Read the model definition and answer for the solid it produces. Units are mm, in the model's axes. A direction names the side the tool comes from. Give positions to 0.01 mm unless a question says otherwise; leave off trailing zeros. Write each loop counter-clockwise with the first axis right and the second up, starting at its lowest first coordinate (ties: lowest second). Pieces come first, ordered by that corner, then holes. Notation, with made-up numbers: M 47.5,43.5 L 80.5,43.5 A20 ccw 80.5,54.5 Z; hole C 55,67 d4. An arc over 180 degrees is marked long. Use a Markdown table: item, result. Add a question column.
Item 1: A cutting plane is placed at B-B on y = -7.5. Determine the outline of the cut face in (x, z), then the cut area to 3 significant figures.
Item 2: A cutting plane is placed at C-C on x = 19. Determine the outline of the cut face in (y, z), then the cut area to 3 significant figures.
Item 3: A cutting plane is placed at A-A on z = 34. Determine the outline of the cut face in (x, y), then the cut area to 3 significant figures.
Item 4: Consider probe 1 along Y at (x, z) = (-1, 11); probe 2 along Z at (x, y) = (9.5, -5); probe 3 along Y at (x, z) = (11.5, 16). Determine where each line is inside the solid, lowest interval first. Write a range as [from, to].
Item 5: Given P1, Ø13.5, axis at x = 33.5, z = -1.5, coming from the -Y side; P2, Ø9, axis at y = 40, z = -5, coming from the +X side; P3, Ø2, axis at x = 12, z = 51.5, coming from the -Y side; P4, Ø8, axis at x = 29, z = 48.5, coming from the -Y side, each flat-ended and moving along its own axis, determine where each tip first touches the part or whether it passes through.
Item 6: For faces 1 (the flat face through (32, 0, 2)), 2 (the flat face through (0, 0, 63.5)), 3 (the flat face through (0, 34, 1)), determine the directions among +Z, -Z, +X, -X, +Y, -Y from which every point of the face is accessible in a straight line to the end or side of a thin tool.
from build123d import *

# Parameters (mm, degrees)
F0_R     = 21.5573937043
F1_DEPTH = 63.5
F3_DEPTH = 1.778
F5_DEPTH = 1.27


with BuildPart() as f1:
    # F0 (on Top) → F1 (new body)
    with BuildSketch(Plane.XY):
        Circle(F0_R)
    extrude(amount=F1_DEPTH)

    # F2 (on Right) → F3 (join)
    with BuildSketch(Plane.YZ):
        with BuildLine():
            add(Edge.make_bspline(
                [(21.4230585843, 18.8257303089), (25.4152571812, 17.7337542467), (35.0627733159, 15.0948933727), (62.3459313723, -26.3349238901), (35.309978925, -8.8714455783), (21.5757172555, 0)],
                knots=[0, 0, 0, 0, 0.257781652, 0.6229531389, 1, 1, 1, 1], degree=3))
            Line((21.4230585843, 18.8257303089), (21.5757172555, 0))
        make_face()
    extrude(amount=F3_DEPTH)

    # F4 (on Front) → F5 (join)
    with BuildSketch(Plane.XZ):
        with BuildLine():
            Line((21.2236842012, 18.8214), (21.2236842012, 0))
            add(Edge.make_bspline(
                [(21.2236842012, 18.8214), (23.8559514528, 18.2657870203), (30.4596483204, 16.8021538854), (61.2280877119, -21.6449576492), (34.4408537462, -5.8542687668), (21.2236842012, 0)],
                knots=[0, 0, 0, 0, 0.2264847707, 0.6174984663, 1, 1, 1, 1], degree=3))
        make_face()
    extrude(amount=F5_DEPTH)


solid = f1.part
Filled in:
| question | item | result |
|---|---|---|
| 1 | outline | M -20.21,0 L 20.21,0 L 20.21,63.5 L -20.21,63.5 Z |
| 1 | area | 2,570 mm² |
| 2 | outline | M -10.18,0 L 10.18,0 L 10.18,63.5 L -10.18,63.5 Z |
| 2 | area | 1,290 mm² |
| 3 | outline | C 0,0 d43.11 |
| 3 | area | 1,460 mm² |
| 4 | probe 1 | [-21.53, 21.53] |
| 4 | probe 2 | [0, 63.5] |
| 4 | probe 3 | [-18.23, 18.23] |
| 5 | P1 | y = -1.27 |
| 5 | P2 | x = 1.78 |
| 5 | P3 | y = -18.54 |
| 5 | P4 | through |
| 6 | face 1 | +Z, -Z, +X, +Y |
| 6 | face 2 | +Z, +X, -X, +Y, -Y |
| 6 | face 3 | +Z, -Z, -X, +Y |
